Answer from the drawing. Dimensions are ordinates in mm from the lowest x, y and z of the part. Round coordinates to 2 decimals unless told otherwise and drop trailing zeros. Order: outer loops, then holes, each group sorted by start corner. A loop starts at its lowest first (then second) coordinate and runs counter-clockwise, first axis right, second up.
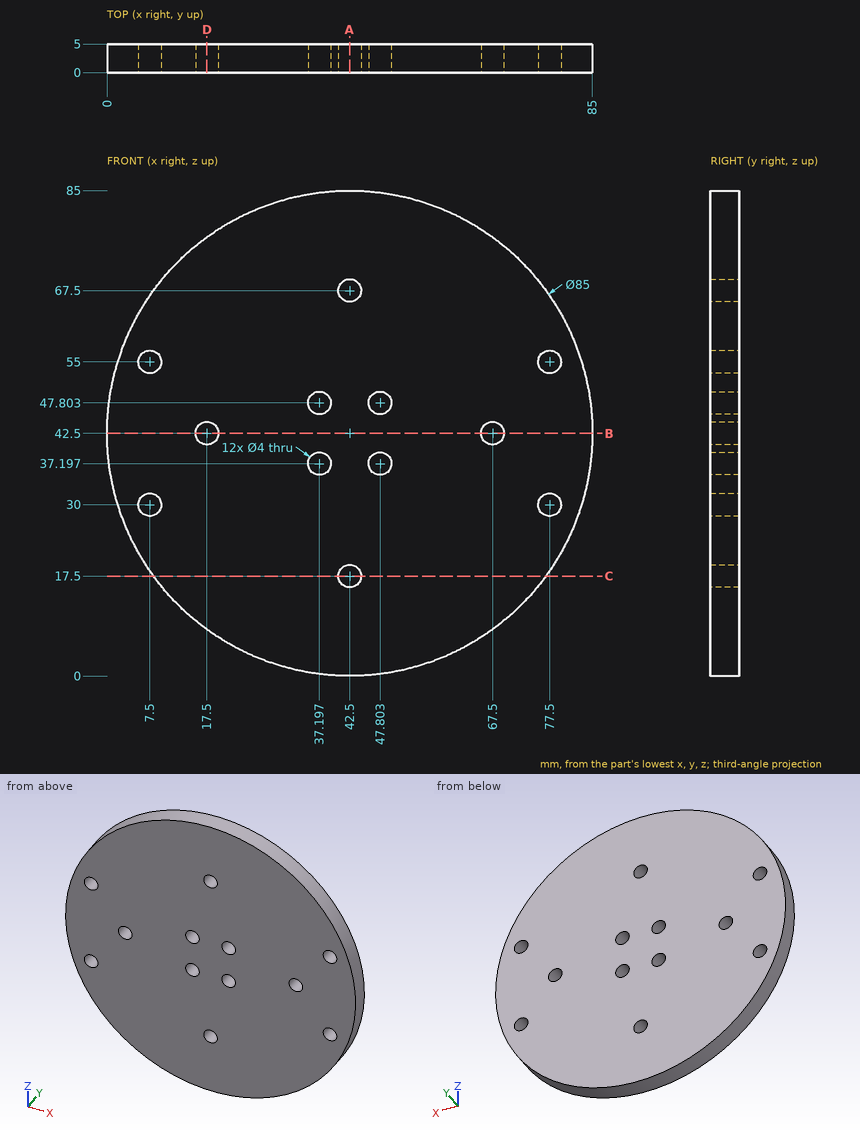
Q1. Straight lines are drawn through the part: probe 1 along Z at (x, y) = (7.5, 1.6); probe 2 along X at (y, z) = (2.05, 41.5); probe 3 along X at (y, z) = (2.55, 30). For each, find the intervals that lie inside material, in ascending order.
Outcome:
probe 1: z = 18.39 to 28, 32 to 53, 57 to 66.61
probe 2: x = 0.01 to 15.77, 19.23 to 65.77, 69.23 to 84.99
probe 3: x = 1.88 to 5.5, 9.5 to 75.5, 79.5 to 83.12
Q2. A cutting plane is placed at D-D, the plane x = 17.5. Give the vertices of the cut face in (y, z), plus the area to 3 significant figures.
Outcome:
outline: (0, 8.13) - (5, 8.13) - (5, 40.5) - (0, 40.5) - close; (0, 44.5) - (5, 44.5) - (5, 76.87) - (0, 76.87) - close
area: 324 mm2
Q3. A cutting plane is placed at B-B, the plane z = 42.5. Give the vertices of the cut face in (x, y).
Outcome:
outline: (0, 0) - (15.5, 0) - (15.5, 5) - (0, 5) - close; (19.5, 0) - (65.5, 0) - (65.5, 5) - (19.5, 5) - close; (69.5, 0) - (85, 0) - (85, 5) - (69.5, 5) - close
Q4. Flat-ended cylindrical pins translate along their axes: pin 1 (6.5 mm diameter, centred on x = 7.5, z = 30, fed in from +Y); pin 2 (2.5 mm diameter, centred on x = 47.8, z = 37.2, fed in from +Y); pin 3 (1.5 mm diameter, centred on x = 39, y = 4.5, fed in from +Z); pin 4 (1.5 mm diameter, centred on y = 1, z = 74, fed in from -X). Find the tip coordinate at first contact, or state that the pin passes through.
Outcome:
pin 1: stops at y = 5
pin 2: passes through
pin 3: stops at z = 84.91
pin 4: stops at x = 13.16
Q5. A cutting plane is placed at A-A, the plane x = 42.5. Give the vertices of the cut face in (y, z).
Outcome:
outline: (0, 0) - (5, 0) - (5, 15.5) - (0, 15.5) - close; (0, 19.5) - (5, 19.5) - (5, 65.5) - (0, 65.5) - close; (0, 69.5) - (5, 69.5) - (5, 85) - (0, 85) - close
Q6. A cutting plane is placed at C-C, the plane z = 17.5. Give the vertices of the cut face in (x, y).
Outcome:
outline: (8.13, 0) - (40.5, 0) - (40.5, 5) - (8.13, 5) - close; (44.5, 0) - (76.87, 0) - (76.87, 5) - (44.5, 5) - close
